Solid Edge part; units mm, degrees
sketch "Sketch1" plane through (0, 0, 0) normal (0, -1, 0) x (1, 0, 0)
  line L0 (-66.0065, -59.7904) -> (33.9935, -59.7904)
  line L1 (33.9935, -59.7904) -> (33.9935, 60.2096)
  line L2 (33.9935, 60.2096) -> (-66.0065, 60.2096)
  line L3 (-66.0065, 60.2096) -> (-66.0065, -59.7904)
  dimension "D1" = 33.9935
  dimension "D2" = 66.0065
extrude "Protrusion1" add sketch "Sketch1" against normal blind 5
sketch "Sketch2" plane through (33.9935, 0, -14.7904) normal (0, -1, 0) x (1, 0, 0)
  circle A0 centre (-20, 55) radius 5
  dimension "D1" = 20
extrude "Cutout1" cut sketch "Sketch2" against normal through all
mirror "Mirror1" about plane through (33.9935, 10, -14.7904) normal (0, 1, 0) of "Protrusion1", "Cutout1"
sketch "Sketch3" plane through (33.9935, 5, -14.7904) normal (0, 1, 0) x (-1, 0, 0)
  line L0 (95, -45) -> (100, -45)
  line L1 (100, -45) -> (100, 75)
  line L2 (100, 75) -> (95, 75)
  line L3 (95, 75) -> (95, -45)
  line L4 (100, -45) -> (60, -45)
  line L5 (60, -45) -> (60, -40)
  line L6 (60, -40) -> (100, -40)
  line L7 (100, -40) -> (100, -45)
  dimension "D1" = 60
  dimension "D2" = 60
  dimension "D3" = 100
  dimension "D4" = 100
  dimension "D5" = 100
extrude "Protrusion3" add sketch "Sketch3" along normal up to surface (10 mm away)
sketch "Sketch4" plane through (33.9935, 10, -59.7904) normal (0, 0, -1) x (-1, 0, 0)
  circle A0 centre (80, 0.1607) radius 7.5
extrude "ExtrudedProtrusion_4" add sketch "Sketch4" along normal blind 10
properties material "Aluminum, 6061-T6"
For this review, take the finished solid that the model builds, in its own axes (mm). A direction names the side the tool comes from. Coordinates: 2 decimals unless noted, no trailing zeros. Order: outer loops, then holes, each group sorted by start corner. A loop starts at its lowest first (then second) coordinate and runs counter-clockwise, first axis right, second up. Notation, with made-up numbers: (4.25, 39) - (61.25, 39) arc R15 cw to (61.25, 48) - close; hole circle Ø4 at (21, -37.75). An arc over 180 degrees is marked (long way). Answer as CSV lines item,"result". Start each with the question number.
1) Draft analysis for pull direction X (two halves, no side actions). For faces 3 (the flat face through (-26.006, 10, -57)), 4 (the cylindrical face through (-38.514, 9.831, -64.72)), 5 (the flat face through (-13, 15, -1)), 6 (the cylindrical face through (10, 2.5, 37.2)), state which applies: +X half, -X half, draft (parallel to the pull), parting line (faces both ways), or undercut.
2) Add section A-A (x = 10.5). State the section outline as (y, z) points.
3) To check wall thickness, follow line 1 along Y through (x, z) = (-41, -38); line 2 along Z through (x, y) = (-55, 4.5); line 3 along X through (y, z) = (7, 53). State the ranges of each line that lie inside material, in increasing order. Write a range as [from, to].
4) Add section B-B (z = -3). State the section outline as (x, y) points, then the cut area to 3 significant figures.
5) Add section D-D (x = -35). State the section outline as (y, z) points, then the cut area to 3 significant figures.
6) Insertion check: P1, Ø3, axis at y = 7.5, z = 23, coming from the +X side; P2, Ø9, axis at x = 13.99, z = 40.21, coming from the +Y side; P3, Ø8, axis at x = -19, y = 5.5, coming from the -Z side; P4, Ø4, axis at y = 9.5, z = -56.5, coming from the +X side. Each pin has a flat end and moves straight along its axis. Give the tip position at first contact, or say it passes through.
7) Machinability: for faces 1 (the flat face through (-66.006, 10, 1)), 2 (the flat face through (-43, 10, -54.79)), which of the approach directions +Z, -Z, +X, -X, +Y, -Y give a long, thin tool a straight path to every point of the face, cutting with its end or side? Answer none if there is none.
8) Add section C-C (x = -20). State the section outline as (y, z) points.
Result:
1,face 3,"+X half"
1,face 4,"parting line"
1,face 5,"draft"
1,face 6,"undercut"
2,outline,"(0, -59.79) - (5, -59.79) - (5, 36.63) - (0, 36.63) - close; (0, 43.79) - (5, 43.79) - (5, 60.21) - (0, 60.21) - close; (15, -59.79) - (20, -59.79) - (20, 36.63) - (15, 36.63) - close; (15, 43.79) - (20, 43.79) - (20, 60.21) - (15, 60.21) - close"
3,line 1,"[0, 5], [15, 20]"
3,line 2,"[-59.79, 60.21]"
3,line 3,"[-66.01, -61.01]"
4,outline,"(-66.01, 0) - (33.99, 0) - (33.99, 5) - (-61.01, 5) - (-61.01, 15) - (33.99, 15) - (33.99, 20) - (-66.01, 20) - close"
4,area,"1,050 mm^2"
5,outline,"(0, -59.79) - (20, -59.79) - (20, 60.21) - (15, 60.21) - (15, -54.79) - (5, -54.79) - (5, 60.21) - (0, 60.21) - close"
5,area,"1,250 mm^2"
6,P1,"x = -61.01"
6,P2,"through"
6,P3,"z = -59.79"
6,P4,"x = -26.01"
7,face 1,"+Z, -Z, -X, +Y, -Y"
7,face 2,"+Z, +X"
8,outline,"(0, -59.79) - (5, -59.79) - (5, 60.21) - (0, 60.21) - close; (15, -59.79) - (20, -59.79) - (20, 60.21) - (15, 60.21) - close"
